Read the model definition and answer for the solid it produces. Units are mm, in the model's axes. Face numbers are marked on the shaded views. Give positions to 0.01 mm unless a question says otherwise; leave off trailing zeros. Write each loop counter-clockwise with the first axis right and the second up, starting at its lowest first coordinate (ties: lowest second). Pieces come first, ordered by that corner, then holes. Notation, with made-up numbers: M 20,13 L 42,13 A15 ccw 42,38 Z; hole C 18.25,-30 d2. An arc over 180 degrees is marked long. Use a Markdown table: item, result. Add a question column.
Item 1: Consider probe 1 along Z at (x, y) = (-1, 2.4); probe 2 along Z at (x, y) = (-1, 2.8); probe 3 along X at (y, z) = (0.55, -0.5). Determine where each line is inside the solid, lowest interval first. Write a range as [from, to].
Item 2: Given P1, Ø10, axis at x = -7.5, z = 11, coming from the -Y side; P2, Ø1.5, axis at x = 2, z = -11, coming from the -Y side; P3, Ø1.5, axis at y = 3, z = -9, coming from the +X side, each flat-ended and moving along its own axis, determine where each tip first touches the part or whether it passes through.
Item 3: A cutting plane is placed at A-A on y = -0.7. Determine the outline of the cut face in (x, z), then the cut area to 3 significant figures.
Item 4: The mould has two halves that part along X. Classify the marked faces 1 and 2: pulls with the +X half, pulls with the -X half, needs draft (parallel to the pull), parting line crosses it, or undercut.
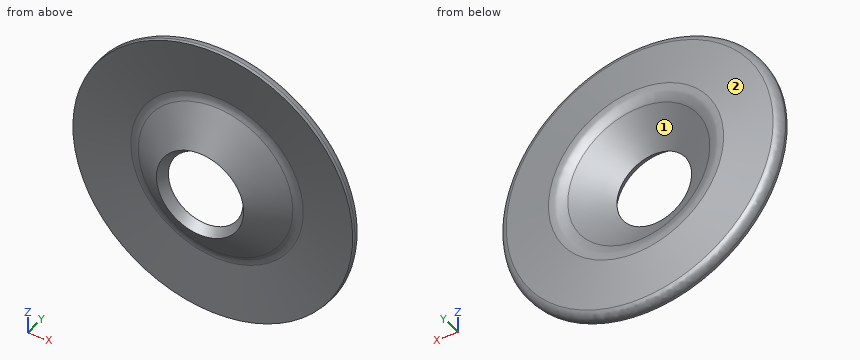
from build123d import *

# Parameters (mm, degrees)
FILLET1_R = 1


with BuildPart() as part:
    # Sketch1 → Revolve-Thin2 (revolve)
    with BuildSketch(Plane.XY, mode=Mode.PRIVATE) as revolve_thin2_sk:
        with BuildLine():
            Line((4.76, 0), (9.049484193, 3.069764451))
            ThreePointArc((9.049484193, 3.069764451), (10.0542655, 3.537150049), (11.160173373, 3.607878762))
            Line((11.160173373, 3.607878762), (18, 2.77))
            Line((18, 2.77), (17.832204304, 1.400239216))
            Line((17.832204304, 1.400239216), (10.992377677, 2.238117978))
            ThreePointArc((10.992377677, 2.238117978), (10.395187426, 2.199924473), (9.85260552, 1.94753625))
            Line((9.85260552, 1.94753625), (5.563121327, -1.122228201))
            Line((5.563121327, -1.122228201), (4.76, 0))
        make_face()
    revolve(revolve_thin2_sk.sketch.rotate(Axis((0, 0, 0), (0, 1, 0)), 90), axis=Axis((0, 0, 0), (0, 1, 0)))

    # Fillet1
    fillet1_edges = [part.edges().sort_by_distance(p)[0] for p in [
        (0, 2.77, 18),
    ]]
    fillet(fillet1_edges, radius=FILLET1_R)


solid = part.part
Filled in:
| question | item | result |
|---|---|---|
| 1 | probe 1 | [-17.72, -8.05], [8.05, 17.72] |
| 1 | probe 2 | [-17.29, -8.61], [8.61, 17.29] |
| 1 | probe 3 | [-7.88, -5.51], [5.51, 7.88] |
| 2 | P1 | y = 0.85 |
| 2 | P2 | y = 2.12 |
| 2 | P3 | x = 15.56 |
| 3 | outline | C 0,0 d12.31; hole C 0,0 d10.52 |
| 3 | area | 32.0 mm² |
| 4 | face 1 | undercut |
| 4 | face 2 | parting line crosses it |
